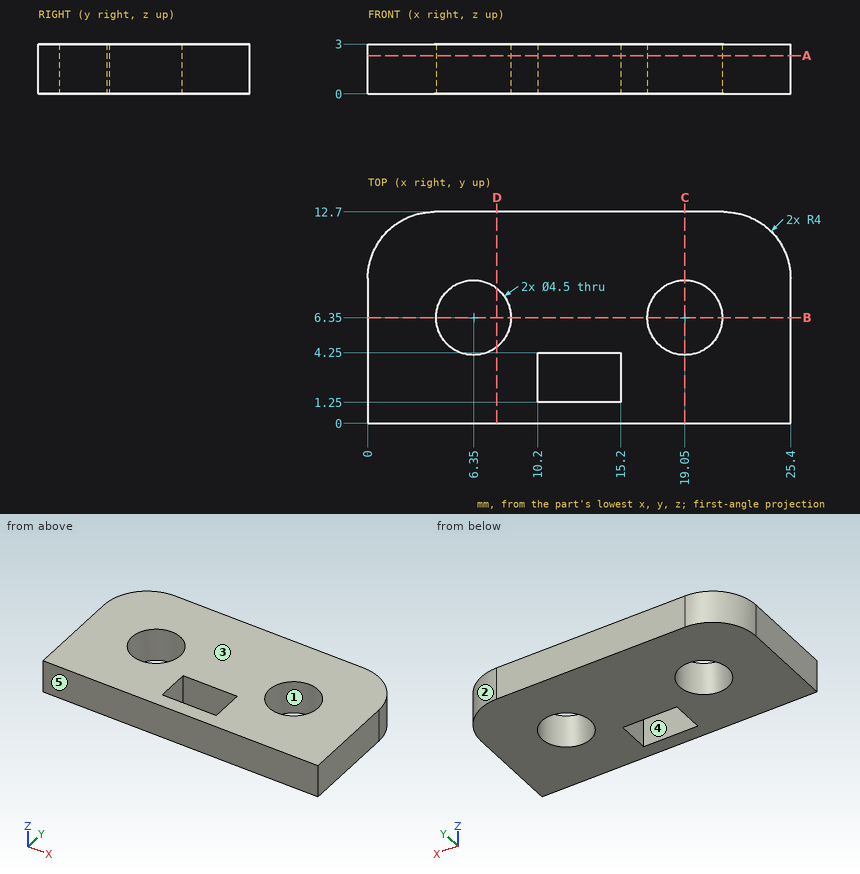
Print and shaded views of the part. All mm, measured from the part's lowest x, y and z. A direction names the side the tool comes from. Round coordinates to 2 decimals unless told otherwise and drop trailing zeros. Write each loop counter-clockwise with the first axis right and the second up, starting at its lowest first coordinate (ties: lowest second). Pieces come first, ordered by that corner, then holes. Notation, with made-up numbers: (56.5, 64) - (104.5, 64) arc R24 cw to (104.5, 77) - close; hole circle Ø5 at (38.25, 31.25). An arc over 180 degrees is marked (long way). One line per item, written item: value.
(1) Cut at B-B, the plane y = 6.35. Give the cut face in (x, z), plus the area to 3 significant figures.
Values follow:
outline: (0, 0) - (4.1, 0) - (4.1, 3) - (0, 3) - close; (8.6, 0) - (16.8, 0) - (16.8, 3) - (8.6, 3) - close; (21.3, 0) - (25.4, 0) - (25.4, 3) - (21.3, 3) - close
area: 49.2 mm²
(2) Cut at C-C, the plane x = 19.05. Give the cut face in (y, z).
Values follow:
outline: (0, 0) - (4.1, 0) - (4.1, 3) - (0, 3) - close; (8.6, 0) - (12.7, 0) - (12.7, 3) - (8.6, 3) - close
(3) Two-plate mould, pull along X, no slides. Class the marked faces 1, 2 and 3: pulls with the +X half, pulls with the -X half, needs draft (parallel to the pull), parting line crosses it, or undercut.
Values follow:
face 1: undercut
face 2: pulls with the +X half
face 3: needs draft
(4) Wall check: probe 1 along X at (y, z) = (6.35, 0.8); probe 2 along Y at (x, z) = (6.35, 2.15); probe 3 along X at (y, z) = (5.5, 0.55). Give the ranges that are in metal, low to high.
Values follow:
probe 1: x = 0 to 4.1, 8.6 to 16.8, 21.3 to 25.4
probe 2: y = 0 to 4.1, 8.6 to 12.7
probe 3: x = 0 to 4.27, 8.43 to 16.97, 21.13 to 25.4
(5) Cut at A-A, the plane z = 2.3. Give the cut face in (x, y), plus the area to 3 significant figures.
Values follow:
outline: (0, 0) - (25.4, 0) - (25.4, 8.7) arc R4 ccw to (21.4, 12.7) - (4, 12.7) arc R4 ccw to (0, 8.7) - close; hole circle Ø4.5 at (6.35, 6.35); hole (10.2, 1.25) - (15.2, 1.25) - (15.2, 4.25) - (10.2, 4.25) - close; hole circle Ø4.5 at (19.05, 6.35)
area: 269 mm²
(6) Cut at D-D, the plane x = 7.75. Give the cut face in (y, z).
Values follow:
outline: (0, 0) - (4.59, 0) - (4.59, 3) - (0, 3) - close; (8.11, 0) - (12.7, 0) - (12.7, 3) - (8.11, 3) - close
(7) 3-axis set-ups, long thin cutter, end or side, ignore diameter. For the marked faces 4 and 5: which of +Z, -Z, +X, -X, +Y, -Y reach the whole face in a straight line?
Values follow:
face 4: +Z, -Z
face 5: +Z, -Z, +X, -X, -Y
(8) Drop flat-ended pins along their axis: P1, Ø4, axis at x = 13.5, y = 3, coming from the -Z side; P2, Ø4, axis at x = 19.05, y = 6.35, coming from the -Z side. Give the stop position or say it passes through.
Values follow:
P1: stops at z = 0
P2: passes through
